Source: CAD feature listing. Evaluate the final solid. Frame: model axes, mm. A direction names the side the tool comes from. Coordinates: 2 decimals unless noted, no trailing zeros. Order: outer loops, then holes, each group sorted by start corner. A loop starts at its lowest first (then second) coordinate and runs counter-clockwise, first axis right, second up.
```python
from build123d import *

# Parameters (mm, degrees)
SKETCH1_R                                           = 9
BOSS_EXTRUDE1_DEPTH                                 = 4
SKETCH2_R                                           = 7
BOSS_EXTRUDE2_DEPTH                                 = 39
CSK_FOR_1_4_FLAT_HEAD_SOCKET_CAP_SCREW1_D           = 6.7564
CSK_FOR_1_4_FLAT_HEAD_SOCKET_CAP_SCREW1_CSINK_D     = 13.4874
CSK_FOR_1_4_FLAT_HEAD_SOCKET_CAP_SCREW1_CSINK_ANGLE = 82
SKETCH6_R                                           = 16
CUT_EXTRUDE1_DEPTH                                  = 1
SKETCH7_R                                           = 4
CUT_EXTRUDE2_DEPTH                                  = 3
SKETCH9_W                                           = 8
SKETCH9_H                                           = 5
CUT_EXTRUDE3_DEPTH                                  = 3
CIRPATTERN1_COUNT                                   = 4
SKETCH10_R                                          = 8
BOSS_EXTRUDE3_DEPTH                                 = 5
SKETCH11_R                                          = 7
CUT_EXTRUDE4_START                                  = -9
SKETCH12_R                                          = 3.3782
CUT_EXTRUDE4_DEPTH                                  = 9


with BuildPart() as part:
    # Sketch1 → Boss-Extrude1 (new body)
    with BuildSketch(Plane.XY):
        Circle(SKETCH1_R)
    extrude(amount=BOSS_EXTRUDE1_DEPTH)

    # Sketch2 → Boss-Extrude2 (add)
    with BuildSketch(Plane.XY.offset(4)):
        Circle(SKETCH2_R)
    extrude(amount=BOSS_EXTRUDE2_DEPTH)

    # CSK for 1/4 Flat Head Socket Cap Screw1 (through all)
    with Locations(Plane.XY.offset(43)):
        with Locations((0, 0)):
            CounterSinkHole(CSK_FOR_1_4_FLAT_HEAD_SOCKET_CAP_SCREW1_D / 2, CSK_FOR_1_4_FLAT_HEAD_SOCKET_CAP_SCREW1_CSINK_D / 2, counter_sink_angle=CSK_FOR_1_4_FLAT_HEAD_SOCKET_CAP_SCREW1_CSINK_ANGLE)

    # Sketch6 → Cut-Extrude1 (cut)
    with BuildSketch(Plane(origin=(0, 0, 0), x_dir=(-1, 0, 0), z_dir=(0, 0, -1))):
        Circle(SKETCH6_R)
    extrude(amount=-CUT_EXTRUDE1_DEPTH, mode=Mode.SUBTRACT)

    # Sketch7 → Cut-Extrude2 (cut)
    with BuildSketch(Plane(origin=(0, 0, 1), x_dir=(-1, 0, 0), z_dir=(0, 0, -1))):
        Circle(SKETCH7_R)
    extrude(amount=-CUT_EXTRUDE2_DEPTH, mode=Mode.SUBTRACT)

    # Sketch9 → Cut-Extrude3 (cut)
    with BuildSketch(Plane(origin=(6, 0, 0), x_dir=(0, 0, -1), z_dir=(1, 0, 0))):
        with Locations((-25.333705971, 0)):
            Rectangle(SKETCH9_W, SKETCH9_H)
    cut_extrude3 = extrude(amount=CUT_EXTRUDE3_DEPTH, mode=Mode.SUBTRACT)

    # CirPattern1: Cut-Extrude3 ×4 about axis
    cirpattern1_axis = Axis((0, 0, 0), (0, 0, 1))
    for i in range(1, CIRPATTERN1_COUNT):
        add(cut_extrude3.rotate(cirpattern1_axis, i * 360 / CIRPATTERN1_COUNT), mode=Mode.SUBTRACT)

    # Sketch10 → Boss-Extrude3 (add)
    with BuildSketch(Plane.XY.offset(4)):
        Circle(SKETCH10_R)
    extrude(amount=BOSS_EXTRUDE3_DEPTH)

    # Sketch11 → section 1 of loft4
    with BuildSketch(Plane.XY.offset(10), mode=Mode.PRIVATE) as loft4_s1:
        Circle(SKETCH11_R)
    # loft up to a face of the part (loft4)
    loft([Face(Wire([part.edges().sort_by_distance((-5.476376847, 5.831749019, 9))[0]])), loft4_s1.sketch])

    # Sketch12 → Cut-Extrude4 (cut)
    with BuildSketch(Plane.XY.offset(10).offset(CUT_EXTRUDE4_START)):
        Circle(SKETCH12_R)
    extrude(amount=CUT_EXTRUDE4_DEPTH, mode=Mode.SUBTRACT)


solid = part.part
```
Q1. Section query B-B on z = 37. Output: boundary loops of the cut face in (x, y), plus the area to 3 significant figures.
Solutions:
outline: circle Ø14 at (0, 0); hole circle Ø6.76 at (0, 0)
area: 118 mm2
Q2. Pull-direction query (X, two-part tool) for faces 5 (the flat face through (-6, 0, 25)), 6 (the flat face through (6.4, 0, 29.334)), 7 (the flat face through (0, 6, 25)); classes: pulls with the +X half, pulls with the -X half, needs draft (parallel to the pull), parting line crosses it, or undercut.
Solutions:
face 5: pulls with the -X half
face 6: needs draft
face 7: undercut
Q3. Set-up query: faces 1 (the cylindrical face through (3.23, -6.21, 26.27)), 2 (the flat face through (3, -2, 4)), 3 (the flat face through (0, 6.4, 29.334)), 4 (the flat face through (0, -6.4, 29.334)). Return all of +Z, -Z, +X, -X, +Y, -Y with unobstructed straight access to the full face (end or side cutting, diameter ignored); none if empty.
Solutions:
face 1: +Z
face 2: -Z
face 3: +Y
face 4: -Y
Q4. Pin query (flat end, axial travel): P1, Ø6, axis at x = -1, z = 19, coming from the +Y side; P2, Ø3, axis at y = 0, z = 7.5, coming from the -X side; P3, Ø5, axis at x = 5, z = 38.5, coming from the -Y side; P4, Ø0.5, axis at x = -0.5, y = 6.5, coming from the +Z side. Return the tip coordinate at first contact, or that it passes through.
Solutions:
P1: stops at y = 7
P2: stops at x = -8
P3: stops at y = -6.54
P4: stops at z = 43
Q5. Material intervals for line 1 along Y through (x, z) = (0.25, 18); line 2 along Y through (x, z) = (0, 2.8); line 3 along X through (y, z) = (0, 26), sorted ascending.
Solutions:
line 1: y = -7 to -3.37, 3.37 to 7
line 2: y = -9 to -4, 4 to 9
line 3: x = -6 to -3.38, 3.38 to 6
